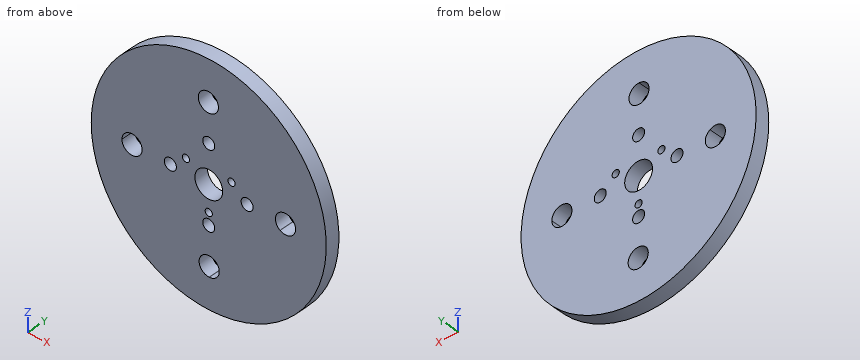
Autodesk Inventor part; units mm, degrees
ref_plane "YZ Plane" through (0, 0, 0) normal (1, 0, 0) x (0, 1, 0)
ref_plane "XZ Plane" through (0, 0, 0) normal (0, 1, 0) x (-1, 0, 0)
ref_plane "XY Plane" through (0, 0, 0) normal (0, 0, 1) x (1, 0, 0)
sketch "Эскиз1" plane through (0, 0, 0) normal (0, 1, 0) x (-1, 0, 0)
  arc A0 (-0.25, 9.2247) -> (0.25, 9.2247) centre (0, 8) ccw
  line L0 (-0.25, 10.9972) -> (-0.25, 9.2247)
  arc A1 (-0.25, 10.9972) -> (-1.1469, -10.94) centre (0, 0) ccw
  line L1 (-1.1469, -10.6297) -> (-1.1469, -10.94)
  line L2 (-0.8473, -10.6297) -> (-1.1469, -10.6297)
  line L3 (-0.8473, -10.9673) -> (-0.8473, -10.6297)
  arc A2 (-0.8473, -10.9673) -> (0.8535, -10.9668) centre (0, 0) ccw
  line L4 (0.8535, -10.6297) -> (0.8535, -10.9668)
  line L5 (1.1541, -10.6297) -> (0.8535, -10.6297)
  line L6 (1.1541, -10.9393) -> (1.1541, -10.6297)
  arc A3 (1.1541, -10.9393) -> (0.25, 10.9972) centre (0, 0) ccw
  line L7 (0.25, 9.2247) -> (0.25, 10.9972)
  circle A4 centre (8, 0) radius 1.25
  circle A5 centre (0, -8) radius 1.25
  circle A6 centre (-8, 0) radius 1.25
  circle A7 centre (0, -5.5) radius 0.75
  circle A8 centre (4.7631, 2.75) radius 0.75
  circle A9 centre (-4.7631, 2.75) radius 0.75
  circle A10 centre (0, 0) radius 2.9
  arc A11 (0.25, 9.2247) -> (-0.25, 9.2247) centre (0, 8) ccw
  circle A12 centre (0, 0) radius 22.5
  point P0 (0, 0)
  dimension "d8" = 45
extrude "Выдавливание1" add sketch "Эскиз1" along normal blind 3 contours A0 L7 A3 L6 L5 L4 A2 L3 L2 L1 A1 L0 | A12
sketch "Эскиз2" plane through (0, 3, 0) normal (0, 1, 0) x (1, 0, 0)
  arc A0 (-14.8717, -1.6857) -> (-18.0997, 0.0968) centre (-15.9998, 0.0856) ccw
  arc A1 (-6.8718, -1.7285) -> (-9.1468, -1.7163) centre (-7.9999, 0.0428) ccw
  circle A2 centre (0, 0) radius 4
  arc A3 (-1.7285, 6.8718) -> (-1.7163, 9.1468) centre (0.0428, 7.9999) ccw
  arc A4 (-1.6857, 14.8717) -> (0.0968, 18.0997) centre (0.0856, 15.9998) ccw
  arc A5 (6.8718, 1.7285) -> (9.1468, 1.7163) centre (7.9999, -0.0428) ccw
  arc A6 (14.8717, 1.6857) -> (18.0997, -0.0968) centre (15.9998, -0.0856) ccw
  arc A7 (1.7285, -6.8718) -> (1.7163, -9.1468) centre (-0.0428, -7.9999) ccw
  arc A8 (1.6857, -14.8717) -> (-0.0968, -18.0997) centre (-0.0856, -15.9998) ccw
  circle A9 centre (-15.9998, 0.0856) radius 2.1
  circle A10 centre (-7.9999, 0.0428) radius 2.1
  circle A11 centre (0, 0) radius 4
  circle A12 centre (0.0428, 7.9999) radius 2.1
  circle A13 centre (0.0856, 15.9998) radius 2.1
  circle A14 centre (7.9999, -0.0428) radius 2.1
  circle A15 centre (15.9998, -0.0856) radius 2.1
  circle A16 centre (-0.0428, -7.9999) radius 2.1
  circle A17 centre (-0.0856, -15.9998) radius 2.1
  dimension "d4" = 4.2
extrude "Выдавливание2" cut sketch "Эскиз2" against normal blind 10 contours A9 A0 | A13 A4 | A15 A6 | A17 A8
offset faces "Размер1" outward 2 faces at (-22.427, 2, -1.8105)
sketch "Эскиз3" plane through (0, 3, 0) normal (0, 1, 0) x (1, 0, 0)
  circle A0 centre (15.9998, -0.0856) radius 2.1
  circle A1 centre (-15.9998, 0.0856) radius 2.1
  circle A2 centre (0.0856, 15.9998) radius 2.1
  circle A3 centre (-0.0856, -15.9998) radius 2.1
  circle A4 centre (0, 0) radius 2.9
  circle A5 centre (8, 0) radius 1.25
  circle A6 centre (0, 8) radius 1.25
  circle A7 centre (-8, 0) radius 1.25
  circle A8 centre (4.7631, -2.75) radius 0.75
  circle A9 centre (-4.7631, -2.75) radius 0.75
  circle A10 centre (0, 5.5) radius 0.75
  circle A11 centre (0, -8) radius 1.25
  circle A12 centre (0, 0) radius 24.5
properties part number "КВ33.044.405 -  Боковина шкива"
Check sheet for the modelled part. Datum: model origin and axes. Units: mm. Round coordinates to 2 decimals unless told otherwise and drop trailing zeros. Order: outer loops, then holes, each group sorted by start corner. A loop starts at its lowest first (then second) coordinate and runs counter-clockwise, first axis right, second up. Notation, with made-up numbers: M 83.5,81.5 L 138.5,81.5 A21 ccw 138.5,115.5 Z; hole C 45,-29.5 d6. An arc over 180 degrees is marked long. Answer in a Markdown table with one row per item.
(1) Gauge pin test, flat end, axial feed: pin 1 (1.5 mm diameter, centred on x = -8, y = 2, fed in from -Z). Record the tip position at first contact, or that the pin passes through.
Findings:
| item | result |
|---|---|
| pin 1 | stops at z = -23.4 |
(2) Section check A-A on z = 8. Record the boundary of the cut face in (x, y).
Findings:
| item | result |
|---|---|
| outline | M -23.16,0 L -1.25,0 L -1.25,3 L -23.16,3 Z; M 1.25,0 L 23.16,0 L 23.16,3 L 1.25,3 Z |
(3) Section check B-B on y = 1.45. Give the number of separate pieces and of enclosed holes in the cut face, plus the area to 3 significant figures.
Findings:
| item | result |
|---|---|
| separate pieces | 1 |
| enclosed holes | 12 |
| area | 1,780 mm^2 |
(4) Section check C-C on x = 8. Record the boundary of the cut face in (y, z), plus the area to 3 significant figures.
Findings:
| item | result |
|---|---|
| outline | M 0,-23.16 L 3,-23.16 L 3,-1.25 L 0,-1.25 Z; M 0,1.25 L 3,1.25 L 3,23.16 L 0,23.16 Z |
| area | 131 mm^2 |
(5) Section check D-D on z = -19.5. Record the boundary of the cut face in (x, y).
Findings:
| item | result |
|---|---|
| outline | M -14.83,0 L 14.83,0 L 14.83,3 L -14.83,3 Z |
(6) Material ranges on line 1 along X through (y, z) = (1.5, 0); line 2 along X through (y, z) = (1.35, 1); line 3 along X through (y, z) = (2.05, -7.5), recorded low to high. Write a range as from..to.
Findings:
| item | result |
|---|---|
| line 1 | x = -24.5..-18.1, -13.9..-9.25, -6.75..-2.9, 2.9..6.75, 9.25..13.9, 18.1..24.5 |
| line 2 | x = -24.48..-17.8, -14.2..-8.75, -7.25..-2.72, 2.72..7.25, 8.75..14.11, 17.89..24.48 |
| line 3 | x = -23.32..-1.15, 1.15..23.32 |
